from build123d import *

# Parameters (mm, degrees)
SKETCH2_W               = 130
SKETCH2_H               = 130
BOSS_EXTRUDE1_DEPTH     = 30
CUT_EXTRUDE1_DEPTH      = 163.102342109
CUT_EXTRUDE1_DEPTH_BACK = 163.102342109
SKETCH3_W               = 20
SKETCH3_H               = 5
CUT_EXTRUDE2_DEPTH      = 163.102342109
CUT_EXTRUDE2_DEPTH_BACK = 163.102342109
SKETCH8_W               = 20
SKETCH8_H               = 5
CUT_EXTRUDE3_DEPTH      = 176.12028954
CUT_EXTRUDE3_DEPTH_BACK = 176.12028954
SKETCH9_R               = 2.5
CUT_EXTRUDE4_DEPTH      = 163.102342109
CUT_EXTRUDE4_DEPTH_BACK = 163.102342109
SKETCH10_W              = 30
SKETCH10_H              = 50
CUT_EXTRUDE5_DEPTH      = 163.102342109
CUT_EXTRUDE5_DEPTH_BACK = 163.102342109
SKETCH12_W              = 5
SKETCH12_H              = 20
CUT_EXTRUDE6_DEPTH      = 10
CUT_EXTRUDE6_DEPTH_BACK = 10
SKETCH13_R              = 2.5


with BuildPart() as part:
    # Sketch2 → Boss-Extrude1 (new body)
    with BuildSketch(Plane(origin=(0, 0, 0), x_dir=(1, 0, 0), z_dir=(0, 1, 0))):
        with Locations((-48.433309961, -46.848350496)):
            Rectangle(SKETCH2_W, SKETCH2_H)
    extrude(amount=BOSS_EXTRUDE1_DEPTH)

    # Sketch3 → Cut-Extrude1 (cut, two sides: drawn at the far end of the back side and taken through both)
    with BuildSketch(Plane(origin=(0, 30, 0), x_dir=(1, 0, 0), z_dir=(0, 1, 0)).offset(-CUT_EXTRUDE1_DEPTH_BACK)):
        with Locations((-103.433309961, 1.151649504)):
            Rectangle(SKETCH3_W, SKETCH3_H)
    extrude(amount=CUT_EXTRUDE1_DEPTH + CUT_EXTRUDE1_DEPTH_BACK, mode=Mode.SUBTRACT)

    # Sketch8 → Cut-Extrude2 (cut, two sides: drawn at the far end of the back side and taken through both)
    with BuildSketch(Plane(origin=(0, 30, 0), x_dir=(1, 0, 0), z_dir=(0, 1, 0)).offset(-CUT_EXTRUDE2_DEPTH_BACK)):
        with Locations((-103.433309961, -30.848350496)):
            Rectangle(SKETCH8_W, SKETCH8_H)
        with Locations((-103.433309961, -62.848350496)):
            Rectangle(SKETCH8_W, SKETCH8_H)
        with Locations((-103.433309961, -94.848350496)):
            Rectangle(SKETCH8_W, SKETCH8_H)
    extrude(amount=CUT_EXTRUDE2_DEPTH + CUT_EXTRUDE2_DEPTH_BACK, mode=Mode.SUBTRACT)

    # Sketch9 → Cut-Extrude3 (cut, two sides: drawn at the far end of the back side and taken through both)
    with BuildSketch(Plane.XY.offset(111.848350496).offset(-CUT_EXTRUDE3_DEPTH_BACK)):
        with Locations((-108.433309961, 14.846459041)):
            Circle(SKETCH9_R)
    extrude(amount=CUT_EXTRUDE3_DEPTH + CUT_EXTRUDE3_DEPTH_BACK, mode=Mode.SUBTRACT)

    # Sketch10 → Cut-Extrude4 (cut, two sides: drawn at the far end of the back side and taken through both)
    with BuildSketch(Plane(origin=(0, 30, 0), x_dir=(1, 0, 0), z_dir=(0, 1, 0)).offset(-CUT_EXTRUDE4_DEPTH_BACK)):
        with Locations((-18.433309961, -6.848350496)):
            Rectangle(SKETCH10_W, SKETCH10_H)
    extrude(amount=CUT_EXTRUDE4_DEPTH + CUT_EXTRUDE4_DEPTH_BACK, mode=Mode.SUBTRACT)

    # Sketch12 → Cut-Extrude5 (cut, two sides: drawn at the far end of the back side and taken through both)
    with BuildSketch(Plane(origin=(0, 30, 0), x_dir=(1, 0, 0), z_dir=(0, 1, 0)).offset(-CUT_EXTRUDE5_DEPTH_BACK)):
        with Locations((-18.433309961, -41.848350496)):
            Rectangle(SKETCH12_W, SKETCH12_H)
    extrude(amount=CUT_EXTRUDE5_DEPTH + CUT_EXTRUDE5_DEPTH_BACK, mode=Mode.SUBTRACT)

    # Sketch13 → Cut-Extrude6 (cut, two sides: drawn at the far end of the back side and taken through both)
    with BuildSketch(Plane(origin=(-20.933309961, 0, 0), x_dir=(0, 0, -1), z_dir=(1, 0, 0)).offset(-CUT_EXTRUDE6_DEPTH_BACK)):
        with Locations(Location((-46.848350496, 12.77430984, 0), (0, 0, 180))):
            Circle(SKETCH13_R)
    extrude(amount=CUT_EXTRUDE6_DEPTH + CUT_EXTRUDE6_DEPTH_BACK, mode=Mode.SUBTRACT)


solid = part.part
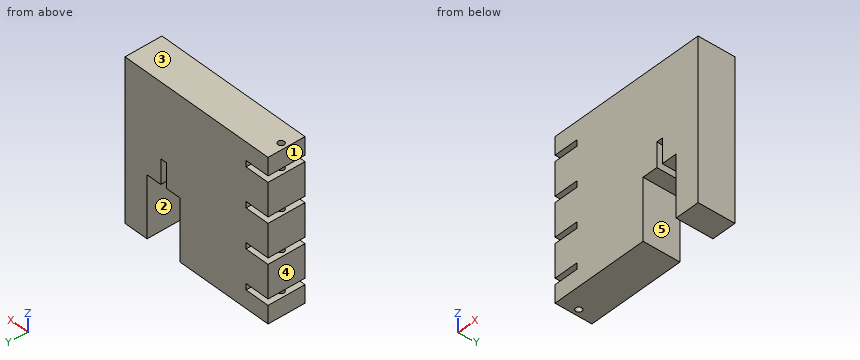
Build history of the part. All positions in model axes, mm. Face numbers are marked on the shaded views. A direction names the side the tool comes from. Coordinates: 2 decimals unless noted, no trailing zeros. Order: outer loops, then holes, each group sorted by start corner. A loop starts at its lowest first (then second) coordinate and runs counter-clockwise, first axis right, second up. Notation, with made-up numbers: (-21, 75.25) - (-13, 75.25) arc R16 cw to (-13, 91.25) - close; hole circle Ø6 at (-31.5, 7.5). An arc over 180 degrees is marked (long way). Put each result on its own line as item: value.
1. Saw through at C-C (y = 19.75). Write the cut outline in (x, z), and give its area (3 significant figures).
Answer sheet:
outline: (-113.43, -18.15) - (-33.43, -18.15) - (-33.43, 31.85) - (-20.93, 31.85) - (-20.93, 51.85) - (-15.93, 51.85) - (-15.93, 31.85) - (-3.43, 31.85) - (-3.43, -18.15) - (16.57, -18.15) - (16.57, 111.85) - (-113.43, 111.85) - (-113.43, 97.35) - (-93.43, 97.35) - (-93.43, 92.35) - (-113.43, 92.35) - (-113.43, 65.35) - (-93.43, 65.35) - (-93.43, 60.35) - (-113.43, 60.35) - (-113.43, 33.35) - (-93.43, 33.35) - (-93.43, 28.35) - (-113.43, 28.35) - (-113.43, 1.35) - (-93.43, 1.35) - (-93.43, -3.65) - (-113.43, -3.65) - close
area: 14,900 mm^2
2. Tool access for the marked faces 4 and 5: list every direction of +Z, -Z, +X, -X, +Y, -Y with a clear straight run to the whole face (end or side of a thin tool).
Answer sheet:
face 4: +Z, -Z, -X, +Y, -Y
face 5: -Z, +Y, -Y
3. Probe line 1 along Z through (x, y) = (-94, 19.5); line 2 along X through (y, z) = (27.25, -8.5); line 3 along X through (y, z) = (20.75, -1). List the from-to ranges inside material, lowest first. Write a range as [from, to].
Answer sheet:
line 1: z = [-18.15, -3.65], [1.35, 28.35], [33.35, 60.35], [65.35, 92.35], [97.35, 111.85]
line 2: x = [-113.43, -33.43], [-3.43, 16.57]
line 3: x = [-93.43, -33.43], [-3.43, 16.57]
4. Pull direction X, two halves, no side cores. Call the marked faces 1, 2 and 3: pulls with the +X half, pulls with the -X half, needs draft (parallel to the pull), parting line crosses it, or undercut.
Answer sheet:
face 1: pulls with the -X half
face 2: undercut
face 3: needs draft
5. Saw through at B-B (z = 10.5). Write the cut outline in (x, y), and give its area (3 significant figures).
Answer sheet:
outline: (-113.43, 0) - (-33.43, 0) - (-33.43, 30) - (-113.43, 30) - close; (-3.43, 0) - (16.57, 0) - (16.57, 30) - (-3.43, 30) - close; hole circle Ø5 at (-108.43, 14.85)
area: 2,980 mm^2
6. Drop flat-ended pins along their axis: P1, Ø1.5, axis at y = 22.5, z = 31.5, coming from the -X side; P2, Ø6, axis at x = -106.5, y = 15, coming from the -Z side; P3, Ø5, axis at x = -8, z = 14, coming from the +Y side; P4, Ø4, axis at x = -18, y = 13.5, coming from the -Z side. Give the stop position or say it passes through.
Answer sheet:
P1: stops at x = -93.43
P2: stops at z = -18.15
P3: passes through
P4: stops at z = 51.85
7. Saw through at A-A (x = -102). Write the cut outline in (y, z), and give its area (3 significant figures).
Answer sheet:
outline: (0, -18.15) - (30, -18.15) - (30, -3.65) - (0, -3.65) - close; (0, 1.35) - (30, 1.35) - (30, 28.35) - (0, 28.35) - close; (0, 33.35) - (30, 33.35) - (30, 60.35) - (0, 60.35) - close; (0, 65.35) - (30, 65.35) - (30, 92.35) - (0, 92.35) - close; (0, 97.35) - (30, 97.35) - (30, 111.85) - (0, 111.85) - close
area: 3,300 mm^2
8. Saw through at D-D (x = -24). Write the cut outline in (y, z), and give its area (3 significant figures).
Answer sheet:
outline: (0, 31.85) - (30, 31.85) - (30, 111.85) - (0, 111.85) - close; hole circle Ø5 at (12.77, 46.85)
area: 2,380 mm^2
